from build123d import *

# Parameters (mm, degrees)
F0_W     = 24.5
F0_H     = 21
F1_DEPTH = 15
F2_T     = -2
F4_DEPTH = 19


with BuildPart() as f1:
    # F0 (on Top) → F1 (new body)
    with BuildSketch(Plane.XY):
        Rectangle(F0_W, F0_H)
    extrude(amount=F1_DEPTH)

    # F2
    f2_openings = [f1.faces().sort_by_distance(p)[0] for p in [
        (0, 0, 0),
        (0, 10.5, 7.5),
    ]]
    offset(amount=F2_T, openings=f2_openings)

    # F3 (on face) → F4 (join)
    with BuildSketch(Plane(origin=(0, -8.5, 0), x_dir=(-1, 0, 0), z_dir=(0, 1, 0))):
        Polygon((-10.25, 2.8284271247), (-10.25, 0), (-8.8357864376, 1.4142135624), align=None)
        Polygon((8.8357864376, 1.4142135624), (10.25, 0), (10.25, 2.8284271247), align=None)
    extrude(amount=F4_DEPTH)


solid = f1.part
Model file for the job. Use its own axes, mm. A direction names the side the tool comes from. Coordinates: 2 decimals unless noted, no trailing zeros. Write each loop counter-clockwise with the first axis right and the second up, starting at its lowest first coordinate (ties: lowest second). Pieces come first, ordered by that corner, then holes. Notation, with made-up numbers: (40, 54) -> (50, 54) arc R24 cw to (50, 67) -> close; hole circle Ø6 at (6, 68.5). An arc over 180 degrees is marked (long way). One line per item, written item: value. Start each with the question number.
1) Pull direction Z, two halves, no side cores. Call faces 4 (the face through (9.53, 0.87, 2.11)), 5 (the face through (12.25, 0, 7)), 6 (the face through (0, 0, 15)): +Z half, -Z half, draft (parallel to the pull), parting line (faces both ways), or undercut.
2) Slice it at C-C on x = 7. Write the cut outline in (y, z), then the cut area to 3 significant figures.
3) Flat gauge pins, fed straight in: pin 1 Ø3 at (x, z) = (5.5, 2.5) entering from +Y; pin 2 Ø1 at (x, y) = (-2.5, -7.5) entering from -Z. Where does each tip first touch, or does it go through?
4) Slice it at B-B on z = 6. Write the cut outline in (x, y), then the cut area to 3 significant figures.
5) Which spindle directions (+Z, -Z, +X, -X, +Y, -Y) get a long thin tool onto all of the face, cutting with end or side? Do faces 1 (the face through (10.25, 1, 8)), 2 (the face through (0, -10.5, 7)), 3 (the face through (9.55, 0.87, 0.7)). Say none if no direction does.
6) Probe probe 1 along X at (y, z) = (-6, 11.25); probe 2 along Y at (x, z) = (-8.5, 11.25); probe 3 along Z at (x, y) = (-1, 1.5). List the from-to ranges inside material, lowest first.
7) Slice it at A-A on y = 5.25. Write the cut outline in (x, z).
Answers follow:
1. face 4: undercut
1. face 5: draft
1. face 6: +Z half
2. outline: (-10.5, 0) -> (-8.5, 0) -> (-8.5, 13) -> (10.5, 13) -> (10.5, 15) -> (-10.5, 15) -> close
2. area: 68.0 mm2
3. pin 1: y = -8.5
3. pin 2: z = 13
4. outline: (-12.25, -10.5) -> (12.25, -10.5) -> (12.25, 10.5) -> (10.25, 10.5) -> (10.25, -8.5) -> (-10.25, -8.5) -> (-10.25, 10.5) -> (-12.25, 10.5) -> close
4. area: 125 mm2
5. face 1: +Y
5. face 2: +Z, -Z, +X, -X, -Y
5. face 3: -Z, +Y
6. probe 1: -12.25 to -10.25, 10.25 to 12.25
6. probe 2: -10.5 to -8.5
6. probe 3: 13 to 15
7. outline: (-12.25, 0) -> (-10.25, 0) -> (-8.84, 1.41) -> (-10.25, 2.83) -> (-10.25, 13) -> (10.25, 13) -> (10.25, 2.83) -> (8.84, 1.41) -> (10.25, 0) -> (12.25, 0) -> (12.25, 15) -> (-12.25, 15) -> close
